Input: dimensioned drawing with shaded views. Units: mm. Origin: part minimum x, y, z. A direction names the side the tool comes from. Give positions to 0.01 mm unless a question says otherwise; leave off trailing zeros. Order: outer loops, then holes, each group sorted by start corner. A loop starts at its lowest first (then second) coordinate and runs counter-clockwise, first axis right, second up.
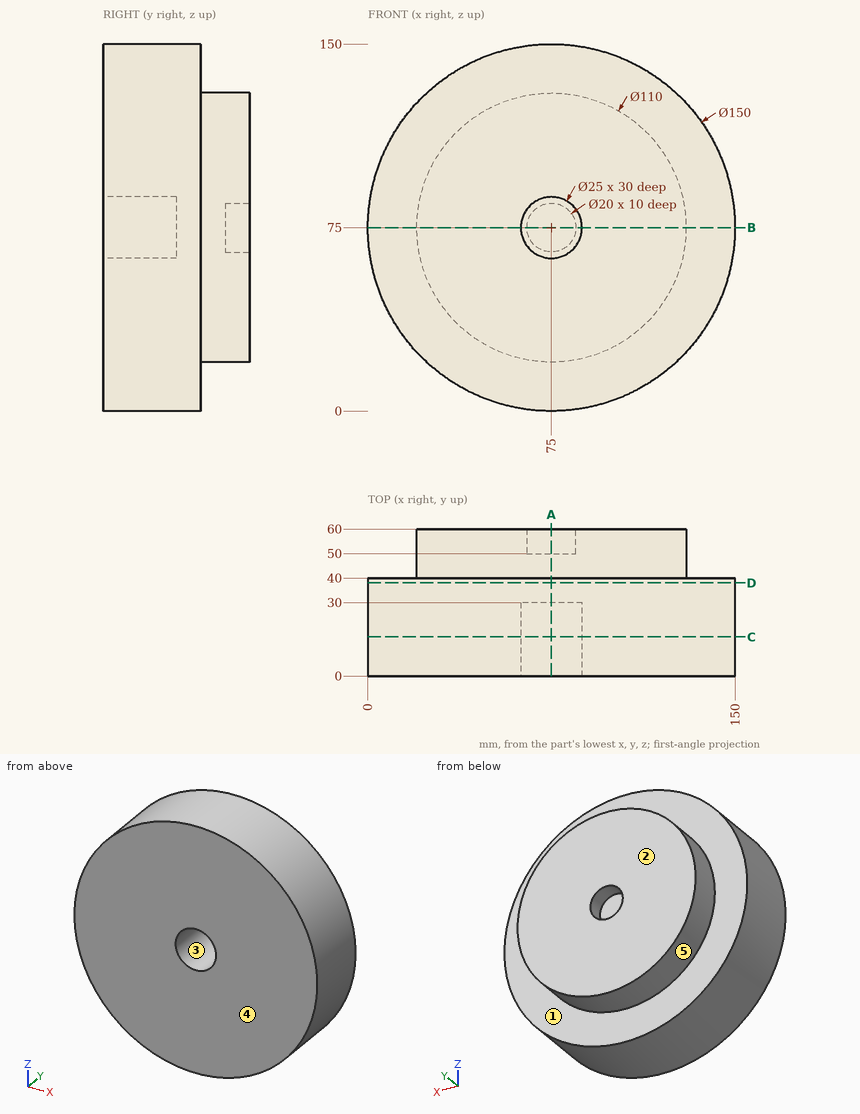
1) Reachability of the marked faces 1 and 2 from +Z, -Z, +X, -X, +Y, -Y: full face, straight path, thin tool, end or side. Return the list, or none.
Report:
face 1: +Y
face 2: +Z, -Z, +X, -X, +Y
2) Material intervals for L1, parallel to Z at x = 75, y = 14.25; L2, parallel to Z at x = 75, y = 55; L3, parallel to Y at x = 133, z = 112, sorted ascending.
Report:
L1: z = 0 to 62.5, 87.5 to 150
L2: z = 20 to 65, 85 to 130
L3: y = 0 to 40
3) Draft query along Z for the marked faces 3, 4 and 5. Return one class per face: +Z half, -Z half, draft (parallel to the pull), parting line (faces both ways), or undercut.
Report:
face 3: undercut
face 4: draft
face 5: parting line
4) Section query D-D, the plane y = 38. Return the cut outline in (x, z), and give its area (3 significant figures).
Report:
outline: circle Ø150 at (75, 75)
area: 17,700 mm2
5) Section query A-A, the plane x = 75. Return the cut outline in (y, z).
Report:
outline: (0, 0) - (40, 0) - (40, 20) - (60, 20) - (60, 65) - (50, 65) - (50, 85) - (60, 85) - (60, 130) - (40, 130) - (40, 150) - (0, 150) - (0, 87.5) - (30, 87.5) - (30, 62.5) - (0, 62.5) - close
6) Section query C-C, the plane y = 16. Return the cut outline in (x, z), and give its area (3 significant figures).
Report:
outline: circle Ø150 at (75, 75); hole circle Ø25 at (75, 75)
area: 17,200 mm2
7) Section query B-B, the plane z = 75. Return the cut outline in (x, y).
Report:
outline: (0, 0) - (62.5, 0) - (62.5, 30) - (87.5, 30) - (87.5, 0) - (150, 0) - (150, 40) - (130, 40) - (130, 60) - (85, 60) - (85, 50) - (65, 50) - (65, 60) - (20, 60) - (20, 40) - (0, 40) - close
8) Pin query (flat end, axial travel): pin 1 (10 mm diameter, centred on x = 77.5, z = 76, fed in from +Y); pin 2 (10 mm diameter, centred on x = 101, y = 6, fed in from +Z); pin 3 (7.5 mm diameter, centred on x = 79, z = 74, fed in from -Y). Return the tip coordinate at first contact, or that it passes through.
Report:
pin 1: stops at y = 50
pin 2: stops at z = 147
pin 3: stops at y = 30
